Verification items for the finished model (mm, model axes). A direction names the side the tool comes from. Round coordinates to 2 decimals unless told otherwise and drop trailing zeros. Write each loop counter-clockwise with the first axis right and the second up, starting at its lowest first coordinate (ties: lowest second). Pieces come first, ordered by that corner, then holes.
Solid Edge part; units mm, degrees
sketch "Sketch1" plane through (0, 0, 0) normal (1, 0, 0) x (0, 1, 0)
  line L0 (133.75, 14.8) -> (-22.25, 14.8)
  line L1 (-22.25, 14.8) -> (-22.25, 11.8)
  line L2 (-22.25, 11.8) -> (-24.25, 11.8)
  line L3 (-24.25, 11.8) -> (-24.25, 9.6)
  line L4 (-24.25, 9.6) -> (-34.75, 9.6)
  line L5 (-34.75, 9.6) -> (-34.75, -0.2)
  line L6 (-34.75, -0.2) -> (-24.25, -0.2)
  line L7 (-24.25, -0.2) -> (146.25, -0.2)
  line L8 (146.25, 9.8) -> (146.25, -0.2)
  line L9 (135.75, 9.8) -> (146.25, 9.8)
  line L10 (135.75, 9.8) -> (135.75, 11.8)
  line L11 (135.75, 11.8) -> (133.75, 11.8)
  line L12 (133.75, 11.8) -> (133.75, 14.8)
revolve "RevolvedProtrusion1" add sketch "Sketch1" angle 360 about axis through (0, -24.25, -0.2) along (0, 1, 0)
sketch "Sketch2" plane through (0, -22.25, 0) normal (0, -1, 0) x (1, 0, 0)
  line L0 (20, -4.2309) -> (20, -16.2309)
  line L1 (20, -16.2309) -> (15, -13.11)
  line L2 (15, -13.11) -> (15, -20)
  line L3 (15, -20) -> (-14.8, -20)
  line L4 (-14.8, -20) -> (-14.8, -13.1132)
  line L5 (-20, -16) -> (-14.8, -13.1132)
  line L6 (-20, -4) -> (-20, -16)
  line L7 (-20, -4) -> (-15, -6.8868)
  line L8 (-15, -6.8868) -> (-15, 0)
  line L9 (-15, 0) -> (15, 0)
  line L10 (15, 0) -> (15, -6.89)
  line L11 (20, -4.2309) -> (15, -6.89)
extrude "Protrusion1" add sketch "Sketch2" against normal blind 15
extrude "Protrusion2" [suppressed]
sketch "Sketch3" plane through (0, 146.25, -0.2) normal (0, 1, 0) x (-1, 0, 0)
  line L0 (6.45, -5.25) -> (6.45, 5.65)
  arc A0 (6.45, 5.65) -> (5.45, 6.65) centre (5.45, 5.65) ccw
  line L1 (5.45, 6.65) -> (-5.45, 6.65)
  arc A1 (-5.45, 6.65) -> (-6.45, 5.65) centre (-5.45, 5.65) ccw
  line L2 (-6.45, 5.65) -> (-6.45, -5.25)
  arc A2 (-5.45, -6.25) -> (-6.45, -5.25) centre (-5.45, -5.25) cw
  line L3 (-5.45, -6.25) -> (5.45, -6.25)
  arc A3 (5.45, -6.25) -> (6.45, -5.25) centre (5.45, -5.25) ccw
extrude "Anschluss1" add sketch "Sketch3" along normal blind 10
sketch "Sketch4" plane through (0, 146.25, -0.2) normal (0, 1, 0) x (-1, 0, 0)
  line L0 (6.45, -5.25) -> (6.45, 5.65)
  arc A0 (6.45, 5.65) -> (5.45, 6.65) centre (5.45, 5.65) ccw
  line L1 (5.45, 6.65) -> (-5.45, 6.65)
  arc A1 (-5.45, 6.65) -> (-6.45, 5.65) centre (-5.45, 5.65) ccw
  line L2 (-6.45, 5.65) -> (-6.45, -5.25)
  arc A2 (-5.45, -6.25) -> (-6.45, -5.25) centre (-5.45, -5.25) cw
  line L3 (-5.45, -6.25) -> (5.45, -6.25)
  arc A3 (5.45, -6.25) -> (6.45, -5.25) centre (5.45, -5.25) ccw
extrude "ExtrudedProtrusion_8" add sketch "Sketch4" against normal blind 190
extrude "Cutout1" [suppressed]
sketch "Sketch5" plane through (15, 55.75, -3.445) normal (1, 0, 0) x (0, 1, 0)
  circle A0 centre (-70.5, 1.445) radius 0.9
extrude "ExtrudedCutout_5" cut sketch "Sketch5" against normal blind 30
sketch "Sketch6" plane through (15, 55.75, -3.445) normal (1, 0, 0) x (0, 1, 0)
  circle A0 centre (70.5, 1.445) radius 0.9
extrude "ExtrudedCutout_6" cut sketch "Sketch6" against normal blind 30
sketch "Sketch7" plane through (15, 55.75, -3.445) normal (1, 0, 0) x (0, 1, 0)
  circle A0 centre (-1, 1.445) radius 0.9
extrude "ExtrudedCutout_7" cut sketch "Sketch7" against normal blind 30
sketch "Sketch8" plane through (0, 133.75, -0.2) normal (0, 1, 0) x (-1, 0, 0)
  line L0 (-20, -4.0309) -> (-20, -16.0309)
  line L1 (-20, -16.0309) -> (-15, -12.91)
  line L2 (-15, -12.91) -> (-15, -19.8)
  line L3 (-15, -19.8) -> (14.8, -19.8)
  line L4 (14.8, -19.8) -> (14.8, -12.9132)
  line L5 (14.8, -12.9132) -> (20, -15.8)
  line L6 (20, -15.8) -> (20, -3.8)
  line L7 (20, -3.8) -> (15, -6.6868)
  line L8 (15, -6.6868) -> (15, 0.2)
  line L9 (15, 0.2) -> (-15, 0.2)
  line L10 (-15, 0.2) -> (-15, -6.69)
  line L11 (-15, -6.69) -> (-20, -4.0309)
extrude "ExtrudedProtrusion_9" add sketch "Sketch8" against normal blind 15
sketch "Sketch9" plane through (15, 55.75, -3.445) normal (1, 0, 0) x (0, 1, 0)
  circle A0 centre (70.5, 1.445) radius 0.9
extrude "ExtrudedCutout_8" cut sketch "Sketch9" against normal blind 30
sketch "Sketch10" plane through (0, 133.75, -0.2) normal (0, 1, 0) x (-1, 0, 0)
  line L0 (-5.1, -10.1993) -> (-5.1, -19.8)
  line L1 (-5.1, -19.8) -> (4.9, -19.8)
  line L2 (4.9, -19.8) -> (4.9, -10.1993)
  line L3 (4.9, -10.1993) -> (-5.1, -10.1993)
extrude "ExtrudedProtrusion_10" add sketch "Sketch10" against normal blind 156
sketch "Sketch11" plane through (0, 133.75, -0.2) normal (0, 1, 0) x (-1, 0, 0)
  line L0 (-10, 17.75) -> (-10, 12.25)
  line L1 (-10, 12.25) -> (10, 12.25)
  line L2 (10, 12.25) -> (10, 17.75)
  line L3 (10, 17.75) -> (-10, 17.75)
extrude "ExtrudedCutout_9" cut sketch "Sketch11" against normal blind 156
sketch "Sketch12" plane through (-12.45, 47.75, -10.1) normal (0, 1, 0) x (-1, 0, 0)
  line L0 (7.55, -5.9) -> (7.55, 6.1)
  line L1 (7.55, 6.1) -> (2.55, 3.2132)
  line L2 (2.55, 3.2132) -> (2.55, 10.1)
  line L3 (2.55, 10.1) -> (-27.45, 10.1)
  line L4 (-27.45, 10.1) -> (-27.45, 3.21)
  line L5 (-27.45, 3.21) -> (-32.45, 5.8691)
  line L6 (-32.45, 5.8691) -> (-32.45, -6.1309)
  line L7 (-32.45, -6.1309) -> (-27.45, -3.01)
  line L8 (-27.45, -3.01) -> (-27.45, -9.9)
  line L9 (-27.45, -9.9) -> (2.35, -9.9)
  line L10 (2.35, -9.9) -> (2.35, -3.0132)
  line L11 (2.35, -3.0132) -> (7.55, -5.9)
extrude "ExtrudedProtrusion_11" add sketch "Sketch12" along normal blind 15
sketch "Sketch13" plane through (15, 55.75, -3.445) normal (1, 0, 0) x (0, 1, 0)
  circle A0 centre (-1, 1.445) radius 0.9
extrude "ExtrudedCutout_10" cut sketch "Sketch13" against normal blind 30
Q1. Depth check by flat-ended pin: P1, Ø1, axis at x = 9, z = -13.5, coming from the +Y side; P2, Ø2, axis at y = -14.75, z = -2, coming from the +X side; P3, Ø8, axis at y = 152.5, z = -2.5, coming from the +X side; P4, Ø5.5, axis at y = 126.5, z = -18.5, coming from the +X side. Enter the tip coordinate at first touch or a pass-through.
Recorded:
P1: stops at y = 133.75
P2: stops at x = 15
P3: stops at x = 6.45
P4: stops at x = 20
Q2. Material ranges on line 1 along Y through (x, z) = (-16.5, -6.5); line 2 along Z through (x, y) = (8, -14.75); line 3 along Y through (x, z) = (-4, -2.5), recorded low to high.
Recorded:
line 1: y = -22.25 to -7.25, 47.75 to 62.75, 118.75 to 133.75
line 2: z = -20 to -2.9, -1.1 to 12.05
line 3: y = -43.75 to -15.5, -14 to 54, 55.5 to 125.5, 127 to 156.25
Q3. Tool access check on faces 1 (the flat face through (-9, -24.25, -5)), 2 (the flat face through (0, 151, 6.45)), 3 (the flat face through (-14.8, 126, -17)), 4 (the flat face through (-4.9, 21, -17)). Record the directions out of +Z, -Z, +X, -X, +Y, -Y that give a thin tool (end or side, any length) a straight path to the whole face; none if there is none.
Recorded:
face 1: -Y
face 2: +Z, +X, -X, +Y
face 3: -Z, +Y, -Y
face 4: -Z, -X
Q4. Sectioned sample at A-A (y = 96.5). Enter the section's corners in (x, z).
Recorded:
outline: (-8.66, 12.05) arc R15 ccw to (-4.9, -14.38) - (-4.9, -20) - (5.1, -20) - (5.1, -14.31) arc R15 ccw to (8.66, 12.05) - close
Q5. Release check for a two-part mould opening along X. For faces 5 (the flat face through (-12, 118.75, -12)), 6 (the cylindrical face through (-0.53, 134.74, -12.19)), 7 (the flat face through (-15, 55.1, -3.5)) record: released by +X, released by -X, zero draft, split by the parting line, or undercut.
Recorded:
face 5: zero draft
face 6: split by the parting line
face 7: undercut
